For this review, take the finished solid that the model builds, in its own axes (mm). A direction names the side the tool comes from. Round coordinates to 2 decimals unless told otherwise and drop trailing zeros. Loops run counter-clockwise (first coordinate to the right, second up) from the corner with the lowest first, then second, coordinate; pieces in that order, holes last. Notation, with made-up numbers: M 55,-11 L 90,-11 A24 ccw 90,6 Z; hole C -8,25 d9. An arc over 180 degrees is marked long. One line per question, with ' | ' between items. Start each with the question number.
1) Mouldability with a two-part tool opening along X and no side actions: class faces 5 (the face through (-7.03, 3, 0.29)), 6 (the face through (-2.7, -3.23, -1.13)), 7 (the face through (12.223, -3.932, 1.135)), 8 (the face through (4, 2, -1.588)) as pulls with the +X half, pulls with the -X half, needs draft (parallel to the pull), parting line crosses it, or undercut.
2) For pin 1 Ø1.5 at (x, y) = (-2.5, 3.5) entering from +Z, flat-tipped, find the tip position at first contact; note if it passes through.
3) We need section A-A (y = -3.75). State how many separate pieces and enclosed holes the cut face has, and give its area (3 significant figures).
4) We need section C-C (z = -0.2). Give the boundary of the cut face in (x, y), and give its area (3 significant figures).
5) For probe 1 along X at (y, z) = (-4, 0) (3 decimals); probe 2 along Y at (x, z) = (8.5, -1.15); probe 3 along X at (y, z) = (-3.25, -0.75), list the stretches that pass through material, from the lowest coordinate up. Write a range as from..to.
6) For faces 1 (the face through (-2.7, -3.23, 1.13)), 2 (the face through (-0.477, 0.023, -1.135)), 3 (the face through (-2.72, 3.18, 1.11)), 4 (the face through (11.135, 2.58, -0.022)), list the 3-axis set-ups (+Z, -Z, +X, -X, +Y, -Y) from which the entire face can be reached by the end or side of a thin tool; tool diameter is ignored.
7) We need section B-B (x = 6.75). Give the boundary of the cut face in (y, z).
```python
from build123d import *

# Parameters (mm, degrees)
F1_DEPTH = 1.5875
F3_DEPTH = 4.445
F4_R     = 1.58749
F5_R     = 1.143
F6_DEPTH = 12.7
F8_DEPTH = 12.7


# Not quite as in the source:
# - a fillet or chamfer is up to 0.001 mm smaller than in the source, because OpenCascade refuses the exact size


with BuildPart() as f1:
    # F0 (on Top) → F1 (new body, symmetric)
    with BuildSketch(Plane.XY):
        Polygon((12.7, 1.651), (12.7, 4.826), (-3.175, 4.826), (-3.175, 1.5875), (-9.525, 1.5875), (-9.525, -1.5875), (-3.175, -1.5875), (-3.175, -4.826), (12.7, -4.826), (12.7, -1.651), (0, -1.651), (0, 0), (0, 1.651), align=None)
    extrude(amount=F1_DEPTH, both=True)

    # F2 (on Front) → F3 (join, symmetric)
    with BuildSketch(Plane.XZ):
        with BuildLine():
            ThreePointArc((-8.89, 0), (-7.9375, -0.9525), (-6.985, 0))
            ThreePointArc((-6.985, 0), (-7.9375, 0.9525), (-8.89, 0))
        make_face()
    extrude(amount=F3_DEPTH, both=True)

    # F4 (radius 1.5875 in the source; OpenCascade refuses exactly that, so slightly less here)
    f4_edges = [f1.edges().sort_by_distance(p)[0] for p in [
        (-3.175, 3.20675, -1.5875),
        (-3.175, 3.20675, 1.5875),
        (-3.175, -3.20675, 1.5875),
        (-3.175, -3.20675, -1.5875),
        (-9.525, 0, 1.5875),
        (-9.525, 0, -1.5875),
        (12.7, 3.2385, -1.5875),
        (12.7, 3.2385, 1.5875),
        (12.7, -3.2385, 1.5875),
        (12.7, -3.2385, -1.5875),
        (0, 0, 1.5875),
        (0, 0, -1.5875),
    ]]
    fillet(f4_edges, radius=F4_R)

    # F5 (on Front) → F6 (cut, symmetric)
    with BuildSketch(Plane.XZ):
        with Locations((9.525, 0)):
            Circle(F5_R)
    extrude(amount=F6_DEPTH, both=True, mode=Mode.SUBTRACT)

    # F7 (on Top) → F8 (cut, symmetric)
    with BuildSketch(Plane.XY):
        Polygon((9.525, 1.651), (9.525, -1.651), (15.875, -5.3171742094), (15.875, 5.3171742094), align=None)
        Polygon((-9.525, 4.445), (-9.525, 3.997129469), (-6.985, 4.445), align=None)
        Polygon((-9.525, -4.445), (-6.985, -4.445), (-9.525, -3.997129469), align=None)
    extrude(amount=F8_DEPTH, both=True, mode=Mode.SUBTRACT)


solid = f1.part
```
Answers below:
1) face 5: undercut | face 6: undercut | face 7: pulls with the +X half | face 8: needs draft
2) pin 1: z = 1.58
3) separate pieces: 2 | enclosed holes: 1 | area: 47.0 mm^2
4) outline: M -9.51,-1.59 L -8.87,-1.59 L -8.87,-4.11 L -7.01,-4.44 L -7.01,-1.59 L -3.16,-1.59 L -3.16,-4.83 L 8.4,-4.83 L 8.4,-1.65 L -0.01,-1.65 L -0.01,1.65 L 8.4,1.65 L 8.4,4.83 L -3.16,4.83 L -3.16,1.59 L -7.01,1.59 L -7.01,4.44 L -8.87,4.11 L -8.87,1.59 L -9.51,1.59 Z; M 10.65,-4.83 L 12.69,-4.83 L 12.69,-3.48 L 10.65,-2.3 Z; M 10.65,2.3 L 12.69,3.48 L 12.69,4.83 L 10.65,4.83 Z | area: 122 mm^2
5) probe 1: -8.89..-6.985, -3.175..8.382, 10.668..12.7 | probe 2: -4.83..-1.65, 1.65..4.83 | probe 3: -8.52..-7.35, -2.99..8.66, 10.39..12.29
6) face 1: +Z, -Y | face 2: -Z, +X | face 3: +Z, +Y | face 4: +Z, -Z, +X
7) outline: M -4.83,-1.59 L -1.65,-1.59 L -1.65,1.59 L -4.83,1.59 Z; M 1.65,-1.59 L 4.83,-1.59 L 4.83,1.59 L 1.65,1.59 Z
